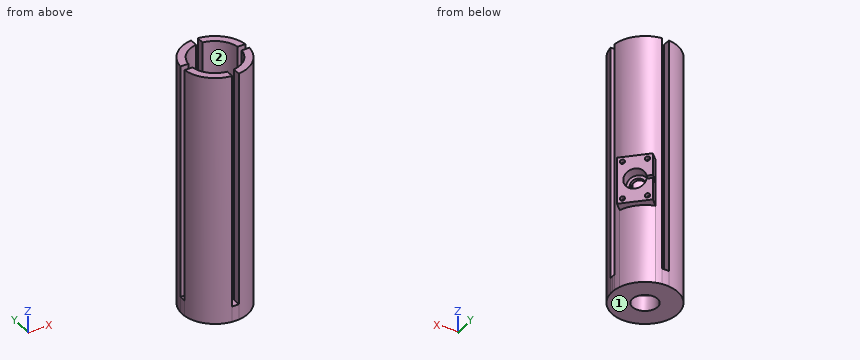
```python
from build123d import *

# Parameters (mm, degrees)
BOSS_EXTRUDE2_DEPTH   = 203.2
BOSS_EXTRUDE2_2_DEPTH = 203.2
BOSS_EXTRUDE2_3_DEPTH = 203.2
BOSS_EXTRUDE2_4_DEPTH = 203.2
SKETCH1_15_R          = 10.16
BOSS_EXTRUDE3_DEPTH   = 12.7
BOSS_EXTRUDE4_DEPTH   = 101.6
CUT_EXTRUDE2_DEPTH    = 63.5
SKETCH4_R             = 8.300000037
CUT_EXTRUDE3_DEPTH    = 8.89
SKETCH5_R             = 5.715
CUT_EXTRUDE5_DEPTH    = 25.4
SKETCH7_W             = 2.54
SKETCH7_H             = 6
CUT_EXTRUDE6_DEPTH    = 8.89
SKETCH8_R             = 1.8542
CUT_EXTRUDE7_DEPTH    = 3.81


with BuildPart() as part:
    # Sketch1 → Boss-Extrude2 (new body)
    with BuildSketch(Plane.XY):
        with BuildLine():
            Line((-26.533104764, 2.69875), (-20.139988789, 2.69875))
            ThreePointArc((-20.139988789, 2.69875), (-14.368409794, 14.368409794), (-2.69875, 20.139988789))
            Line((-2.69875, 20.139988789), (-2.69875, 26.533104764))
            ThreePointArc((-2.69875, 26.533104764), (-18.858537854, 18.858537854), (-26.533104764, 2.69875))
        make_face()
    extrude(amount=BOSS_EXTRUDE2_DEPTH)



with BuildPart() as body_2:
    # Sketch1 → Boss-Extrude2 2 (new body)
    with BuildSketch(Plane.XY):
        with BuildLine():
            ThreePointArc((-2.69875, -20.139988789), (-14.368409794, -14.368409794), (-20.139988789, -2.69875))
            Line((-20.139988789, -2.69875), (-26.533104764, -2.69875))
            ThreePointArc((-26.533104764, -2.69875), (-18.858537854, -18.858537854), (-2.69875, -26.533104764))
            Line((-2.69875, -26.533104764), (-2.69875, -20.139988789))
        make_face()
    extrude(amount=BOSS_EXTRUDE2_2_DEPTH)


with BuildPart() as body_3:
    # Sketch1 → Boss-Extrude2 3 (new body)
    with BuildSketch(Plane.XY):
        with BuildLine():
            Line((2.69875, 26.533104764), (2.69875, 20.139988789))
            ThreePointArc((2.69875, 20.139988789), (14.368409794, 14.368409794), (20.139988789, 2.69875))
            Line((20.139988789, 2.69875), (26.533104764, 2.69875))
            ThreePointArc((26.533104764, 2.69875), (18.858537854, 18.858537854), (2.69875, 26.533104764))
        make_face()
    extrude(amount=BOSS_EXTRUDE2_3_DEPTH)


with BuildPart() as body_4:
    # Sketch1 → Boss-Extrude2 4 (new body)
    with BuildSketch(Plane.XY):
        with BuildLine():
            ThreePointArc((20.139988789, -2.69875), (14.368409794, -14.368409794), (2.69875, -20.139988789))
            Line((2.69875, -20.139988789), (2.69875, -26.533104764))
            ThreePointArc((2.69875, -26.533104764), (18.858537854, -18.858537854), (26.533104764, -2.69875))
            Line((26.533104764, -2.69875), (20.139988789, -2.69875))
        make_face()
    extrude(amount=BOSS_EXTRUDE2_4_DEPTH)


with BuildPart() as part_1:
    add(part.part)

    add(body_2.part)  # Boss-Extrude3 merges body 2

    add(body_3.part)  # Boss-Extrude3 merges body 3

    add(body_4.part)  # Boss-Extrude3 merges body 4
    # Sketch1_15 → Boss-Extrude3 (add)
    with BuildSketch(Plane.XY):
        with BuildLine():
            Line((-15.24, -2.69875), (-15.24, 2.69875))
            Line((-15.24, 2.69875), (-20.139988789, 2.69875))
            ThreePointArc((-20.139988789, 2.69875), (-20.32, 0), (-20.139988789, -2.69875))
            Line((-20.139988789, -2.69875), (-15.24, -2.69875))
        make_face()
        with BuildLine():
            ThreePointArc((2.69875, 20.139988789), (0, 20.32), (-2.69875, 20.139988789))
            Line((-2.69875, 20.139988789), (-2.69875, 15.24))
            Line((-2.69875, 15.24), (2.69875, 15.24))
            Line((2.69875, 15.24), (2.69875, 20.139988789))
        make_face()
        with BuildLine():
            ThreePointArc((20.32, 0), (20.274947253, 1.352373432), (20.139988789, 2.69875))
            Line((20.139988789, 2.69875), (15.24, 2.69875))
            Line((15.24, 2.69875), (15.24, -2.69875))
            Line((15.24, -2.69875), (20.139988789, -2.69875))
            ThreePointArc((20.139988789, -2.69875), (20.274947253, -1.352373432), (20.32, 0))
        make_face()
        with BuildLine():
            Line((-2.69875, -15.24), (-2.69875, -20.139988789))
            ThreePointArc((-2.69875, -20.139988789), (0, -20.32), (2.69875, -20.139988789))
            Line((2.69875, -20.139988789), (2.69875, -15.24))
            Line((2.69875, -15.24), (-2.69875, -15.24))
        make_face()
        with BuildLine():
            ThreePointArc((20.139988789, -2.69875), (14.368409794, -14.368409794), (2.69875, -20.139988789))
            Line((2.69875, -20.139988789), (2.69875, -26.533104764))
            ThreePointArc((2.69875, -26.533104764), (18.858537854, -18.858537854), (26.533104764, -2.69875))
            Line((26.533104764, -2.69875), (20.139988789, -2.69875))
        make_face()
        with BuildLine():
            ThreePointArc((-2.69875, -20.139988789), (-14.368409794, -14.368409794), (-20.139988789, -2.69875))
            Line((-20.139988789, -2.69875), (-26.533104764, -2.69875))
            ThreePointArc((-26.533104764, -2.69875), (-18.858537854, -18.858537854), (-2.69875, -26.533104764))
            Line((-2.69875, -26.533104764), (-2.69875, -20.139988789))
        make_face()
        with BuildLine():
            Line((-26.533104764, 2.69875), (-20.139988789, 2.69875))
            ThreePointArc((-20.139988789, 2.69875), (-14.368409794, 14.368409794), (-2.69875, 20.139988789))
            Line((-2.69875, 20.139988789), (-2.69875, 26.533104764))
            ThreePointArc((-2.69875, 26.533104764), (-18.858537854, 18.858537854), (-26.533104764, 2.69875))
        make_face()
        with BuildLine():
            Line((2.69875, 26.533104764), (2.69875, 20.139988789))
            ThreePointArc((2.69875, 20.139988789), (14.368409794, 14.368409794), (20.139988789, 2.69875))
            Line((20.139988789, 2.69875), (26.533104764, 2.69875))
            ThreePointArc((26.533104764, 2.69875), (26.163391474, 5.173571938), (25.56336349, 7.602851248))
            Line((25.56336349, 7.602851248), (25.144717139, 7.184204897))
            Line((25.144717139, 7.184204897), (7.184204897, 25.144717139))
            Line((7.184204897, 25.144717139), (7.602851248, 25.56336349))
            ThreePointArc((7.602851248, 25.56336349), (5.173571938, 26.163391474), (2.69875, 26.533104764))
        make_face()
        with BuildLine():
            ThreePointArc((25.56336349, 7.602851248), (18.858537854, 18.858537854), (7.602851248, 25.56336349))
            Line((7.602851248, 25.56336349), (7.184204897, 25.144717139))
            Line((7.184204897, 25.144717139), (25.144717139, 7.184204897))
            Line((25.144717139, 7.184204897), (25.56336349, 7.602851248))
        make_face()
        with BuildLine():
            Line((-20.139988789, 2.69875), (-15.24, 2.69875))
            Line((-15.24, 2.69875), (-15.24, -2.69875))
            Line((-15.24, -2.69875), (-20.139988789, -2.69875))
            ThreePointArc((-20.139988789, -2.69875), (-14.368409794, -14.368409794), (-2.69875, -20.139988789))
            Line((-2.69875, -20.139988789), (-2.69875, -15.24))
            Line((-2.69875, -15.24), (2.69875, -15.24))
            Line((2.69875, -15.24), (2.69875, -20.139988789))
            ThreePointArc((2.69875, -20.139988789), (14.368409794, -14.368409794), (20.139988789, -2.69875))
            Line((20.139988789, -2.69875), (15.24, -2.69875))
            Line((15.24, -2.69875), (15.24, 2.69875))
            Line((15.24, 2.69875), (20.139988789, 2.69875))
            ThreePointArc((20.139988789, 2.69875), (14.368409794, 14.368409794), (2.69875, 20.139988789))
            Line((2.69875, 20.139988789), (2.69875, 15.24))
            Line((2.69875, 15.24), (-2.69875, 15.24))
            Line((-2.69875, 15.24), (-2.69875, 20.139988789))
            ThreePointArc((-2.69875, 20.139988789), (-14.368409794, 14.368409794), (-20.139988789, 2.69875))
        make_face()
        Circle(SKETCH1_15_R, mode=Mode.SUBTRACT)
        with BuildLine():
            Line((-2.69875, 26.533104764), (-2.69875, 20.139988789))
            ThreePointArc((-2.69875, 20.139988789), (0, 20.32), (2.69875, 20.139988789))
            Line((2.69875, 20.139988789), (2.69875, 26.533104764))
            ThreePointArc((2.69875, 26.533104764), (0, 26.67), (-2.69875, 26.533104764))
        make_face()
        with BuildLine():
            ThreePointArc((-20.139988789, -2.69875), (-20.32, 0), (-20.139988789, 2.69875))
            Line((-20.139988789, 2.69875), (-26.533104764, 2.69875))
            ThreePointArc((-26.533104764, 2.69875), (-26.67, 0), (-26.533104764, -2.69875))
            Line((-26.533104764, -2.69875), (-20.139988789, -2.69875))
        make_face()
        with BuildLine():
            ThreePointArc((2.69875, -20.139988789), (0, -20.32), (-2.69875, -20.139988789))
            Line((-2.69875, -20.139988789), (-2.69875, -26.533104764))
            ThreePointArc((-2.69875, -26.533104764), (0, -26.67), (2.69875, -26.533104764))
            Line((2.69875, -26.533104764), (2.69875, -20.139988789))
        make_face()
        with BuildLine():
            Line((26.533104764, 2.69875), (20.139988789, 2.69875))
            ThreePointArc((20.139988789, 2.69875), (20.274947253, 1.352373432), (20.32, 0))
            ThreePointArc((20.32, 0), (20.274947253, -1.352373432), (20.139988789, -2.69875))
            Line((20.139988789, -2.69875), (26.533104764, -2.69875))
            ThreePointArc((26.533104764, -2.69875), (26.635754204, -1.351109902), (26.67, 0))
            ThreePointArc((26.67, 0), (26.635754204, 1.351109902), (26.533104764, 2.69875))
        make_face()
    extrude(amount=BOSS_EXTRUDE3_DEPTH)

    # Sketch1_18 → Boss-Extrude4 (add)
    with BuildSketch(Plane.XY):
        with BuildLine():
            Line((13.470384182, 31.430896424), (7.602851248, 25.56336349))
            ThreePointArc((7.602851248, 25.56336349), (18.858537854, 18.858537854), (25.56336349, 7.602851248))
            Line((25.56336349, 7.602851248), (31.430896424, 13.470384182))
            Line((31.430896424, 13.470384182), (13.470384182, 31.430896424))
        make_face()
    extrude(amount=BOSS_EXTRUDE4_DEPTH)

    # Sketch1_19 → Cut-Extrude2 (cut)
    with BuildSketch(Plane.XY):
        with BuildLine():
            Line((13.470384182, 31.430896424), (7.602851248, 25.56336349))
            ThreePointArc((7.602851248, 25.56336349), (18.858537854, 18.858537854), (25.56336349, 7.602851248))
            Line((25.56336349, 7.602851248), (31.430896424, 13.470384182))
            Line((31.430896424, 13.470384182), (13.470384182, 31.430896424))
        make_face()
    extrude(amount=CUT_EXTRUDE2_DEPTH, mode=Mode.SUBTRACT)

    # Sketch4 → Cut-Extrude3 (cut)
    with BuildSketch(Plane(origin=(22.450640303, 22.450640303, 0), x_dir=(0, 0, -1), z_dir=(0.707106781, 0.707106781, 0))):
        with Locations((-82.55, 0)):
            Circle(SKETCH4_R)
    extrude(amount=-CUT_EXTRUDE3_DEPTH, mode=Mode.SUBTRACT)

    # Sketch5 → Cut-Extrude5 (cut)
    with BuildSketch(Plane(origin=(22.450640303, 22.450640303, 0), x_dir=(0, 0, -1), z_dir=(0.707106781, 0.707106781, 0))):
        with Locations((-82.55, 0)):
            Circle(SKETCH5_R)
    extrude(amount=-CUT_EXTRUDE5_DEPTH, mode=Mode.SUBTRACT)

    # Sketch7 → Cut-Extrude6 (cut)
    with BuildSketch(Plane(origin=(-8.980256121, 8.980256121, 0), x_dir=(0, 0, 1), z_dir=(-0.707106781, 0.707106781, 0))):
        with Locations((82.55, 28.75)):
            Rectangle(SKETCH7_W, SKETCH7_H)
    extrude(amount=-CUT_EXTRUDE6_DEPTH, mode=Mode.SUBTRACT)

    # Sketch8 → Cut-Extrude7 (cut)
    with BuildSketch(Plane(origin=(22.450640303, 22.450640303, 0), x_dir=(0, 0, -1), z_dir=(0.707106781, 0.707106781, 0))):
        with Locations((-97.79, -8.89)):
            Circle(SKETCH8_R)
        with Locations((-97.79, 8.89)):
            Circle(SKETCH8_R)
        with Locations((-67.31, 8.89)):
            Circle(SKETCH8_R)
        with Locations((-67.31, -8.89)):
            Circle(SKETCH8_R)
    extrude(amount=-CUT_EXTRUDE7_DEPTH, mode=Mode.SUBTRACT)


solid = part_1.part
```
Geometry: final body of the model. Coordinates: model frame, mm. Face numbers are marked on the shaded views. Round coordinates to 2 decimals unless told otherwise and drop trailing zeros. Loops run counter-clockwise (first coordinate to the right, second up) from the corner with the lowest first, then second, coordinate; pieces in that order, holes last. Notation, with made-up numbers: (28, 41.25) -> (39, 41.25) arc R18 ccw to (39, 63.25) -> close; hole circle Ø7 at (49, 51.5). An arc over 180 degrees is marked (long way). Write each question's results on one line, items separated by ' | '.
Item 1: Cut plane A-A on z = 109. Return the cut outline in (x, y).
Answers below:
outline: (-26.53, -2.7) arc R26.67 ccw to (-2.7, -26.53) -> (-2.7, -20.14) arc R20.32 cw to (-20.14, -2.7) -> close; (-26.53, 2.7) -> (-20.14, 2.7) arc R20.32 cw to (-2.7, 20.14) -> (-2.7, 26.53) arc R26.67 ccw to start; (2.7, -26.53) arc R26.67 ccw to (26.53, -2.7) -> (20.14, -2.7) arc R20.32 cw to (2.7, -20.14) -> close; (2.7, 20.14) arc R20.32 cw to (20.14, 2.7) -> (26.53, 2.7) arc R26.67 ccw to (2.7, 26.53) -> close
Item 2: Cut plane B-B on x = -7.5. Return the cut outline in (y, z), and give its area (3 significant figures).
Answers below:
outline: (-25.59, 0) -> (-6.85, 0) -> (-6.85, 12.7) -> (-18.89, 12.7) -> (-18.89, 203.2) -> (-25.59, 203.2) -> close; (6.85, 0) -> (25.59, 0) -> (25.59, 203.2) -> (18.89, 203.2) -> (18.89, 12.7) -> (6.85, 12.7) -> close | area: 3,030 mm²
Item 3: Pin query (flat end, axial travel): pin 1 Ø8 at (x, z) = (20, 138) entering from +Y; pin 2 Ø3 at (y, z) = (25, 127) entering from +X; pin 3 Ø3 at (y, z) = (5.5, 160.5) entering from -X. Return the tip coordinate at first contact, or that it passes through.
Answers below:
pin 1: stops at y = 21.34 | pin 2: stops at x = 12.61 | pin 3: stops at x = -26.37
Item 4: Pull-direction query (Y, two-part tool) for the marked faces 1 and 2; classes: pulls with the +Y half, pulls with the -Y half, needs draft (parallel to the pull), parting line crosses it, or undercut.
Answers below:
face 1: needs draft | face 2: undercut
Item 5: Line query: probe 1 along Y at (x, z) = (0, 9.25); probe 2 along Z at (x, y) = (12, 10.5); probe 3 along Z at (x, y) = (18.5, 13). Output: solid intervals per line, ascending. Write a range as [from, to].
Answers below:
probe 1: y = [-26.67, -10.16], [10.16, 26.67] | probe 2: z = [0, 12.7] | probe 3: z = [0, 78.36], [86.74, 203.2]
Item 6: Cut plane C-C on x = -18. Return the cut outline in (y, z), and give its area (3 significant figures).
Answers below:
outline: (-19.68, 0) -> (19.68, 0) -> (19.68, 203.2) -> (9.43, 203.2) -> (9.43, 12.7) -> (-9.43, 12.7) -> (-9.43, 203.2) -> (-19.68, 203.2) -> close | area: 4,410 mm²
